Check sheet for the modelled part. Datum: model origin and axes. Units: mm. A direction names the side the tool comes from. Round coordinates to 2 decimals unless told otherwise and drop trailing zeros. Loops run counter-clockwise (first coordinate to the right, second up) from the corner with the lowest first, then second, coordinate; pieces in that order, holes last. Notation, with made-up numbers: (51, 38.5) - (79, 38.5) arc R10 ccw to (79, 52.5) - close; hole circle Ø11 at (87.5, -27.5). An arc over 180 degrees is marked (long way). Put each result on its own line as item: value.
```python
from build123d import *

# Parameters (mm, degrees)
SKETCH1_W           = 44.45
SKETCH1_H           = 3.175
CHAMFER1_SIZE       = 0.9525
CUT_EXTRUDE2_DEPTH  = 2.86258
BOSS_EXTRUDE2_START = -17.623191003
SKETCH9_R           = 3.175
BOSS_EXTRUDE2_DEPTH = 17.623191003


with BuildPart() as part:
    # Sketch1 → Revolve1 (revolve)
    with BuildSketch(Plane(origin=(0, 0, 0), x_dir=(0, 0, -1), z_dir=(1, 0, 0))):
        with Locations((22.225, 1.5875)):
            Rectangle(SKETCH1_W, SKETCH1_H)
    revolve(axis=Axis((0, 0, -44.45), (0, 0, 1)))

    # Chamfer1
    chamfer1_edges = [part.edges().sort_by_distance(p)[0] for p in [
        (0, -3.175, -44.45),
    ]]
    chamfer(chamfer1_edges, length=CHAMFER1_SIZE)

    # Sketch7 → Revolve2 (revolve)
    with BuildSketch(Plane(origin=(0, 0, 0), x_dir=(0, 0, -1), z_dir=(1, 0, 0)), mode=Mode.PRIVATE) as revolve2_sk:
        with BuildLine():
            Line((0, 6.7437), (0.20447, 6.7437))
            Line((0.20447, 6.7437), (4.0894, 3.366581874))
            ThreePointArc((4.0894, 3.366581874), (4.328282675, 3.224461616), (4.601808997, 3.175))
            Line((4.601808997, 3.175), (4.601808997, 0))
            Line((4.601808997, 0), (0, 0))
            Line((0, 0), (0, 6.7437))
        make_face()
    revolve(revolve2_sk.sketch.rotate(Axis((0, 0, 0), (0, 0, -1)), 180), axis=Axis((0, 0, 0), (0, 0, -1)))

    # Boss-Extrude1 cone 1 section (through the dimple's axis) → Boss-Extrude1 (revolve)
    with BuildSketch(Plane(origin=(0, 0, -4.601808997), x_dir=(0, -1, 0), z_dir=(1, 0, 0))):
        Polygon((0, 0), (3.175, 0), (0, 3.06606186), align=None)
    revolve(axis=Axis((0, 0, -4.601808997), (0, 0, -1)))

    # Sketch5 → Cut-Extrude2 (cut)
    with BuildSketch(Plane.XY):
        Polygon((0, 2.291358881), (-1.984375, 1.14567944), (-1.984375, -1.14567944), (0, -2.291358881), (1.984375, -1.14567944), (1.984375, 1.14567944), align=None)
    extrude(amount=-CUT_EXTRUDE2_DEPTH, mode=Mode.SUBTRACT)

    # Cut-Extrude3 cone 1 section (through the dimple's axis) → Cut-Extrude3 (revolve, cut)
    with BuildSketch(Plane(origin=(0, 0, 0), x_dir=(0, -1, 0), z_dir=(1, 0, 0))):
        Polygon((0, 0), (2.291358881, 0), (0, 1.322916667), align=None)
    revolve(axis=Axis((0, 0, 0), (0, 0, -1)), mode=Mode.SUBTRACT)

    # Sketch9 → Boss-Extrude2 (add)
    with BuildSketch(Plane.XY.offset(-4.601808997).offset(BOSS_EXTRUDE2_START)):
        with Locations(Location((0, 0, 0), (0, 0, 90))):
            Circle(SKETCH9_R)
    extrude(amount=BOSS_EXTRUDE2_DEPTH)


solid = part.part
```
Item 1: Go/stop test with flat-tipped pins: pin 1 (5 mm diameter, centred on y = -1, z = -26, fed in from -X) (3 decimals); pin 2 (1.5 mm diameter, centred on x = 3, y = -0.5, fed in from +Z); pin 3 (2 mm diameter, centred on x = 2, y = 4, fed in from -Z); pin 4 (5 mm diameter, centred on y = -5, z = -23.5, fed in from +X). Record where each tip stops, or that it passes through.
Filled sheet:
pin 1: x = -3.175
pin 2: z = 0
pin 3: z = -3.97
pin 4: x = 1.96
Item 2: Tool access check on faces 1 (the flat face through (1.01, 1.71, -1.41)), 2 (the flat face through (0, 0, -44.45)), 3 (the cylindrical face through (3.1, -0.69, -24.32)). Record the directions out of +Z, -Z, +X, -X, +Y, -Y that give a thin tool (end or side, any length) a straight path to the whole face; none if there is none.
Filled sheet:
face 1: +Z
face 2: -Z, +X, -X, +Y, -Y
face 3: -Z
Item 3: Thickness scan on line 1 (X direction, y = 0, z = -38) (3 decimals); line 2 (Z direction, x = 0, y = 1). Record the ranges inside material, lowest first. Write a range as from..to.
Filled sheet:
line 1: -3.175..3.175
line 2: -44.45..-2.86
Item 4: Release check for a two-part mould opening along Y. For faces 4 (the flat face through (-0.978, 1.727, -1.411)), 5 (the flat face through (0, 3, 0)), 6 (the conical face through (3.13, -1.63, -3.9)) record: +Y half, -Y half, draft (parallel to the pull), parting line (faces both ways), or undercut.
Filled sheet:
face 4: undercut
face 5: draft
face 6: parting line
Item 5: Section check B-B on z = -30. Enter the section's corners in (x, y) (3 decimals), then the cut area to 3 significant figures.
Filled sheet:
outline: circle Ø6.35 at (0, 0)
area: 31.7 mm²
